Geometry check sheet. Reference: the model listing, model coordinates, mm. A direction names the side the tool comes from. Coordinates: 2 decimals unless noted, no trailing zeros. Loops run counter-clockwise (first coordinate to the right, second up) from the corner with the lowest first, then second, coordinate; pieces in that order, holes last. Notation, with made-up numbers: M 58.25,48 L 107.25,48 A29 ccw 107.25,72 Z; hole C 30.5,-6.5 d2. An arc over 180 degrees is marked long. Use CSV: the item, a comma, the result in double quotes.
```python
from build123d import *

# Parameters (mm, degrees)
SKETCH1_W           = 47
SKETCH1_H           = 47
BOSS_EXTRUDE1_DEPTH = 1
SKETCH2_W           = 47
SKETCH2_H           = 47
SKETCH2_W_2         = 45
SKETCH2_H_2         = 45
BOSS_EXTRUDE2_DEPTH = 7.5
SKETCH4_R           = 0.5
CUT_EXTRUDE3_DEPTH  = 1
LPATTERN1_COUNT     = 6
LPATTERN1_PITCH     = 3
FILLET1_R           = 1.5
SKETCH8_W           = 5
SKETCH8_H           = 5
CUT_EXTRUDE4_DEPTH  = 5
BOSS_EXTRUDE3_REACH = 68.312
SKETCH9_R           = 1


with BuildPart() as part:
    # Sketch1 → Boss-Extrude1 (new body)
    with BuildSketch(Plane(origin=(0, 0, 0), x_dir=(1, 0, 0), z_dir=(0, 1, 0))):
        with Locations((23.5, 23.5)):
            Rectangle(SKETCH1_W, SKETCH1_H)
    extrude(amount=BOSS_EXTRUDE1_DEPTH)

    # Sketch2 → Boss-Extrude2 (add)
    with BuildSketch(Plane(origin=(0, 1, 0), x_dir=(1, 0, 0), z_dir=(0, 1, 0))):
        with Locations((23.5, 23.5)):
            Rectangle(SKETCH2_W, SKETCH2_H)
        with Locations((23.5, 23.5)):
            Rectangle(SKETCH2_W_2, SKETCH2_H_2, mode=Mode.SUBTRACT)
    extrude(amount=BOSS_EXTRUDE2_DEPTH)

    # Sketch4 → Cut-Extrude3 (cut)
    with BuildSketch(Plane(origin=(47, 0, 0), x_dir=(0, 0, -1), z_dir=(1, 0, 0))):
        with Locations((16, 2)):
            Circle(SKETCH4_R)
    cut_extrude3 = extrude(amount=-CUT_EXTRUDE3_DEPTH, mode=Mode.SUBTRACT)

    # LPattern1: Cut-Extrude3 ×6
    with Locations(*[(0, 0, -i * LPATTERN1_PITCH) for i in range(1, LPATTERN1_COUNT)]):
        add(cut_extrude3, mode=Mode.SUBTRACT)

    # Fillet1
    fillet1_edges = [part.edges().sort_by_distance(p)[0] for p in [
        (0, 4.25, -47),
        (47, 4.25, -47),
        (47, 4.25, 0),
        (0, 4.25, 0),
    ]]
    fillet(fillet1_edges, radius=FILLET1_R)

    # Sketch8 → Cut-Extrude4 (cut)
    with BuildSketch(Plane.ZY):
        with Locations((-41, 2.5)):
            Rectangle(SKETCH8_W, SKETCH8_H)
        with Locations((-6, 2.5)):
            Rectangle(SKETCH8_W, SKETCH8_H)
    extrude(amount=-CUT_EXTRUDE4_DEPTH, mode=Mode.SUBTRACT)

    # Sketch9 → Boss-Extrude3 (add, up to next)
    with BuildSketch(Plane.XY.offset(-46), mode=Mode.PRIVATE) as boss_extrude3_sk1:
        with Locations(Location((3, 3, 0), (0, 0, 180))):
            Circle(SKETCH9_R)
    boss_extrude3_tool1 = extrude(boss_extrude3_sk1.sketch, amount=BOSS_EXTRUDE3_REACH, mode=Mode.PRIVATE) - part.part
    add(boss_extrude3_tool1.solids().sort_by_distance((3, 3, -46))[0])


solid = part.part
```
1. Release check for a two-part mould opening along Z. For faces 4 (the flat face through (23, 5, -1)), 5 (the flat face through (47, 4, -23)), 6 (the cylindrical face through (46.55, 4.31, -0.43)) record: +Z half, -Z half, draft (parallel to the pull), parting line (faces both ways), or undercut.
The answers:
face 4,"undercut"
face 5,"draft"
face 6,"+Z half"
2. Section check D-D, the plane x = 3. Record the cut outline in (y, z).
The answers:
outline,"M 0,-47 L 8.5,-47 L 8.5,-46 L 4,-46 L 4,-1 L 8.5,-1 L 8.5,0 L 0,0 L 0,-3.5 L 1,-3.5 L 1,-1 L 2,-1 L 2,-46 L 1,-46 L 1,-43.5 L 0,-43.5 Z; M 0,-38.5 L 1,-38.5 L 1,-8.5 L 0,-8.5 Z"
3. Section check B-B, the plane y = 6.5. Record the cut outline in (x, z).
The answers:
outline,"M 0,-45.5 A1.5 ccw 1.5,-47 L 45.5,-47 A1.5 ccw 47,-45.5 L 47,-1.5 A1.5 ccw 45.5,0 L 1.5,0 A1.5 ccw 0,-1.5 Z; hole M 1,-46 L 46,-46 L 46,-1 L 1,-1 Z"
4. Gauge pin test, flat ends, axial feed: P1, Ø22.5, axis at x = 16.5, z = -25, coming from the +Y side; P2, Ø1.1, axis at y = 0.5, z = -40.5, coming from the -X side; P3, Ø1.1, axis at x = 0.5, z = -41, coming from the -Y side. Record the tip position at first contact, or that the pin passes through.
The answers:
P1,"y = 1"
P2,"x = 5"
P3,"y = 5"
5. Set-up check for faces 1 (the flat face through (0.8, 1.4, -8.5)), 2 (the cylindrical face through (0.43, 4.31, -0.45)), 3 (the flat face through (46, 5, -23)): record each of +Z, -Z, +X, -X, +Y, -Y from which the full face is reachable in a straight line by a thin tool's end or side.
The answers:
face 1,"-X, -Y"
face 2,"+Z, -X, +Y, -Y"
face 3,"+Y"
6. Section check A-A, the plane z = -40.5. Record the cut outline in (x, y), plus the area to 3 significant figures.
The answers:
outline,"M 0,5 L 1,5 L 1,8.5 L 0,8.5 Z; C 3,3 d2; M 5,0 L 47,0 L 47,8.5 L 46,8.5 L 46,1 L 5,1 Z"
area,"56.1 mm^2"
7. Section check C-C, the plane z = -11. Record the cut outline in (x, y).
The answers:
outline,"M 0,0 L 47,0 L 47,8.5 L 46,8.5 L 46,1 L 1,1 L 1,8.5 L 0,8.5 Z; C 3,3 d2"
8. Thickness scan on line 1 (X direction, y = 6, z = -40); line 2 (Z direction, x = 6.5, y = 1.25); line 3 (Y direction, x = 46.45, z = -16). Record the ranges inside material, lowest first. Write a range as [from, to].
The answers:
line 1,"[0, 1], [46, 47]"
line 2,"[-47, -46], [-1, 0]"
line 3,"[0, 1.5], [2.5, 8.5]"
